from build123d import *

# Parameters (mm, degrees)
BOSS_EXTRUDE1_DEPTH     = 38.1
SKETCH3_R               = 3.175
BOSS_EXTRUDE3_DEPTH     = 19.05
CUT_EXTRUDE1_DEPTH      = 39.418677326
CUT_EXTRUDE1_DEPTH_BACK = 39.418677326
SKETCH4_R               = 0.79375
CUT_EXTRUDE4_DEPTH      = 8.636
SKETCH6_OUTSIDE_W       = 20.904
SKETCH6_OUTSIDE_H       = 20.248
SKETCH6_OUTSIDE_R       = 2.667
CUT_EXTRUDE5_DEPTH      = 0.762


with BuildPart() as part:
    # Sketch1 → Boss-Extrude1 (new body)
    with BuildSketch(Plane(origin=(0, 0, 0), x_dir=(0, 0, -1), z_dir=(1, 0, 0))):
        Polygon((2.105028301, -3.00161443), (3.651988499, 0.32220077), (1.546960198, 3.323815199), (-2.105028301, 3.00161443), (-3.651988499, -0.32220077), (-1.546960198, -3.323815199), align=None)
    extrude(amount=BOSS_EXTRUDE1_DEPTH)

    # Sketch3 → Boss-Extrude3 (add)
    with BuildSketch(Plane.ZY):
        with Locations(Location((0, 0, 0), (0, 0, 204.958070598))):
            Circle(SKETCH3_R)
    extrude(amount=BOSS_EXTRUDE3_DEPTH)

    # Sketch4 → Cut-Extrude1 (cut, two sides: drawn at the far end of the back side and taken through both)
    with BuildSketch(Plane(origin=(0, 0, 0), x_dir=(1, 0, 0), z_dir=(0, 1, 0)).offset(-CUT_EXTRUDE1_DEPTH_BACK)):
        with Locations(Location((-16.51, 0, 0), (0, 0, 90))):
            Circle(SKETCH4_R)
    extrude(amount=CUT_EXTRUDE1_DEPTH + CUT_EXTRUDE1_DEPTH_BACK, mode=Mode.SUBTRACT)

    # Sketch5 → Cut-Extrude4 (cut)
    with BuildSketch(Plane(origin=(38.1, 0, 0), x_dir=(0, 0, -1), z_dir=(1, 0, 0))):
        with BuildLine():
            Line((-2.878508392, 1.339706848), (-2.105028301, 3.00161443))
            ThreePointArc((-2.105028301, 3.00161443), (-3.323815199, 1.546960198), (-3.651988499, -0.32220077))
            Line((-3.651988499, -0.32220077), (-2.878508392, 1.339706848))
        make_face()
        with BuildLine():
            Line((-2.878508392, 1.339706848), (-3.651988499, -0.32220077))
            Line((-3.651988499, -0.32220077), (-2.599474334, -1.823008005))
            ThreePointArc((-2.599474334, -1.823008005), (-3.162714814, -0.279034054), (-2.878508392, 1.339706848))
        make_face()
        with BuildLine():
            ThreePointArc((-3.651988499, -0.32220077), (-3.00161443, -2.105028301), (-1.546960198, -3.323815199))
            Line((-1.546960198, -3.323815199), (-2.599474334, -1.823008005))
            Line((-2.599474334, -1.823008005), (-3.651988499, -0.32220077))
        make_face()
        with BuildLine():
            Line((-2.599474334, -1.823008005), (-1.546960198, -3.323815199))
            Line((-1.546960198, -3.323815199), (0.279034067, -3.162714813))
            ThreePointArc((0.279034067, -3.162714813), (-1.339706811, -2.878508409), (-2.599474334, -1.823008005))
        make_face()
        with BuildLine():
            ThreePointArc((-1.546960198, -3.323815199), (0.32220077, -3.651988499), (2.105028301, -3.00161443))
            Line((2.105028301, -3.00161443), (0.279034067, -3.162714813))
            Line((0.279034067, -3.162714813), (-1.546960198, -3.323815199))
        make_face()
        with BuildLine():
            Line((0.279034067, -3.162714813), (2.105028301, -3.00161443))
            Line((2.105028301, -3.00161443), (2.878508392, -1.339706848))
            ThreePointArc((2.878508392, -1.339706848), (1.823007983, -2.59947435), (0.279034067, -3.162714813))
        make_face()
        with BuildLine():
            ThreePointArc((2.105028301, -3.00161443), (3.252555442, -1.69166085), (3.666174209, 0))
            ThreePointArc((3.666174209, 0), (3.662626065, 0.16125645), (3.651988499, 0.32220077))
            Line((3.651988499, 0.32220077), (2.878508392, -1.339706848))
            Line((2.878508392, -1.339706848), (2.105028301, -3.00161443))
        make_face()
        with BuildLine():
            Line((2.878508392, -1.339706848), (3.651988499, 0.32220077))
            Line((3.651988499, 0.32220077), (2.599474407, 1.823007901))
            ThreePointArc((2.599474407, 1.823007901), (3.027701789, 0.955848774), (3.175, 0))
            ThreePointArc((3.175, 0), (3.09999106, -0.686061534), (2.878508392, -1.339706848))
        make_face()
        with BuildLine():
            Line((2.599474407, 1.823007901), (3.651988499, 0.32220077))
            ThreePointArc((3.651988499, 0.32220077), (3.00161443, 2.105028301), (1.546960198, 3.323815199))
            Line((1.546960198, 3.323815199), (2.599474407, 1.823007901))
        make_face()
        with BuildLine():
            Line((2.599474407, 1.823007901), (1.546960198, 3.323815199))
            Line((1.546960198, 3.323815199), (-0.279034067, 3.162714813))
            ThreePointArc((-0.279034067, 3.162714813), (1.339706869, 2.878508382), (2.599474407, 1.823007901))
        make_face()
        with BuildLine():
            Line((-0.279034067, 3.162714813), (1.546960198, 3.323815199))
            ThreePointArc((1.546960198, 3.323815199), (-0.32220077, 3.651988499), (-2.105028301, 3.00161443))
            Line((-2.105028301, 3.00161443), (-0.279034067, 3.162714813))
        make_face()
        with BuildLine():
            Line((-0.279034067, 3.162714813), (-2.105028301, 3.00161443))
            Line((-2.105028301, 3.00161443), (-2.878508392, 1.339706848))
            ThreePointArc((-2.878508392, 1.339706848), (-1.823007983, 2.59947435), (-0.279034067, 3.162714813))
        make_face()
    extrude(amount=-CUT_EXTRUDE4_DEPTH, mode=Mode.SUBTRACT)

    # Sketch6 outside → Cut-Extrude5 (cut)
    with BuildSketch(Plane(origin=(36.83, 0, 0), x_dir=(0, 0, -1), z_dir=(1, 0, 0))):
        Rectangle(SKETCH6_OUTSIDE_W, SKETCH6_OUTSIDE_H)
        with Locations(Location((0, 0, 0), (0, 0, 180))):
            Circle(SKETCH6_OUTSIDE_R, mode=Mode.SUBTRACT)
    extrude(amount=CUT_EXTRUDE5_DEPTH, mode=Mode.SUBTRACT)


solid = part.part
The model under review builds one solid part; all positions refer to its coordinate system, in mm. A direction names the side the tool comes from. Coordinates: 2 decimals unless noted, no trailing zeros. Loops run counter-clockwise (first coordinate to the right, second up) from the corner with the lowest first, then second, coordinate; pieces in that order, holes last. Notation, with made-up numbers: (82.25, 64.5) -> (119.25, 64.5) arc R31 cw to (119.25, 96.5) -> close; hole circle Ø2 at (-1, 87). An arc over 180 degrees is marked (long way). Use a Markdown table: item, result. Add a question column.
1. Add section B-B on x = -16.51. Write out the cut boundary in (y, z) (3 decimals), plus the area to 3 significant figures.
2. Add section A-A on x = 2. Write out the cut boundary in (y, z).
3. To check wall thickness, follow line 1 (X direction, y = 0.25, z = 0); line 2 (Z direction, x = -16.51, y = -0.25); line 3 (X direction, y = 1, z = 0.25). State the ranges of each line that lie inside material, in increasing order.
4. Draft analysis for pull direction Z (two halves, no side actions). For faces 4 (the face through (29.464, -0.23, 3.32)), 5 (the face through (-15.735, -0.044, 0.172)), 6 (the face through (14.526, 3.165, 0.253)), state which applies: pulls with the +Z half, pulls with the -Z half, needs draft (parallel to the pull), parting line crosses it, or undercut.
5. Machinability: for faces 1 (the face through (-9.392, -2.142, -2.343)), 2 (the face through (29.464, -2.7, -2)), 3 (the face through (36.83, 2, 2)), which of the approach directions +Z, -Z, +X, -X, +Y, -Y give a long, thin tool a straight path to every point of the face, cutting with its end or side? Answer none if there is none.
6. Clearance check with flat-ended pins moving along their axes: pin 1 Ø3 at (x, y) = (-11.5, -2) entering from -Z; pin 2 Ø1 at (x, y) = (28, -2) entering from +Z; pin 3 Ø2.5 at (x, z) = (-16.51, 0) entering from -Y (3 decimals). State where each tip first meets the part, or that it passes through.
Returned:
| question | item | result |
|---|---|---|
| 1 | outline | (-3.074, -0.794) arc R3.175 ccw to (3.074, -0.794) -> close; (-3.074, 0.794) -> (3.074, 0.794) arc R3.175 ccw to start |
| 1 | area | 21.7 mm² |
| 2 | outline | (-3.32, 1.55) -> (-3, -2.11) -> (0.32, -3.65) -> (3.32, -1.55) -> (3, 2.11) -> (-0.32, 3.65) -> close |
| 3 | line 1 | x = -19.05 to -17.3, -15.72 to 38.1 |
| 3 | line 2 | z = -3.17 to -0.79, 0.79 to 3.17 |
| 3 | line 3 | x = -19.05 to -17.26, -15.76 to 38.1 |
| 4 | face 4 | needs draft |
| 4 | face 5 | undercut |
| 4 | face 6 | pulls with the +Z half |
| 5 | face 1 | -X |
| 5 | face 2 | -Z, +X, -Y |
| 5 | face 3 | none |
| 6 | pin 1 | stops at z = -3.14 |
| 6 | pin 2 | stops at z = 2.83 |
| 6 | pin 3 | stops at y = -3.175 |
